```python
from build123d import *

# Parameters (mm, degrees)
SKETCH1_R           = 2
BOSS_EXTRUDE1_DEPTH = 2
SKETCH2_R           = 0.5
BOSS_EXTRUDE2_DEPTH = 12
DOME1_FACE_RADIUS   = 2
DOME1_HEIGHT        = 0.8
CUT_EXTRUDE1_DEPTH  = 3.8
CIRPATTERN1_COUNT   = 40


with BuildPart() as part:
    # Sketch1 → Boss-Extrude1 (new body)
    with BuildSketch(Plane(origin=(0, 0, 0), x_dir=(0, 0, -1), z_dir=(1, 0, 0))):
        Circle(SKETCH1_R)
    extrude(amount=BOSS_EXTRUDE1_DEPTH)

    # Sketch2 → Boss-Extrude2 (add)
    with BuildSketch(Plane(origin=(2, 0, 0), x_dir=(0, 0, -1), z_dir=(1, 0, 0))):
        Circle(SKETCH2_R)
    extrude(amount=BOSS_EXTRUDE2_DEPTH)

    # Dome1: a dome of height H over a round flat face of radius A is a cap of a sphere of radius (A * A + H * H) / (2 * H)
    dome1_r = (DOME1_FACE_RADIUS * DOME1_FACE_RADIUS + DOME1_HEIGHT * DOME1_HEIGHT) / (2 * DOME1_HEIGHT)
    dome1_base = Plane((0, 0, 0), z_dir=(-1, 0, 0))
    with Locations(dome1_base.offset(DOME1_HEIGHT - dome1_r)):
        dome1_ball = Sphere(dome1_r, mode=Mode.PRIVATE)
    add(split(dome1_ball, bisect_by=dome1_base, keep=Keep.TOP, mode=Mode.PRIVATE))

    # Sketch3 → Cut-Extrude1 (cut, through all)
    with BuildSketch(Plane(origin=(2, 0, 0), x_dir=(0, 0, -1), z_dir=(1, 0, 0))):
        with BuildLine():
            Line((-0.005039775, 1.853565527), (0.135996541, 1.995370878))
            ThreePointArc((0.135996541, 1.995370878), (-0.005437904, 1.999992607), (-0.146845126, 1.994601842))
            Line((-0.146845126, 1.994601842), (-0.005039775, 1.853565527))
        make_face()
    cut_extrude1 = extrude(amount=-CUT_EXTRUDE1_DEPTH, mode=Mode.SUBTRACT)

    # CirPattern1: Cut-Extrude1 ×40 about axis
    cirpattern1_axis = Axis((0, 0, 0), (1, 0, 0))
    for i in range(1, CIRPATTERN1_COUNT):
        add(cut_extrude1.rotate(cirpattern1_axis, i * 360 / CIRPATTERN1_COUNT), mode=Mode.SUBTRACT)


solid = part.part
```
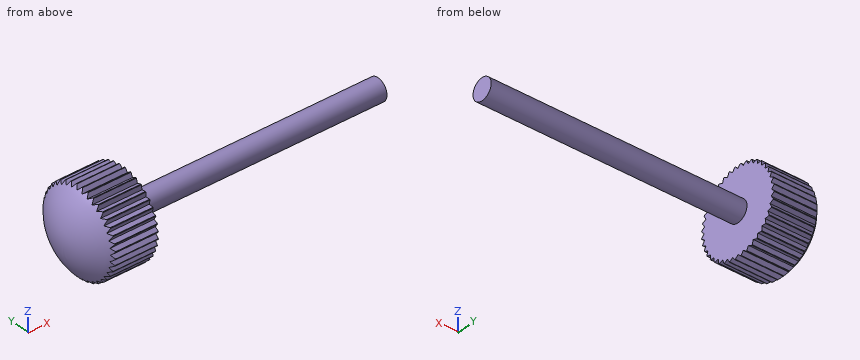
CAD build for the part. Positions are in the model's coordinates, mm. Give positions to 0.01 mm unless a question says otherwise; leave off trailing zeros. Loops run counter-clockwise (first coordinate to the right, second up) from the corner with the lowest first, then second, coordinate; pieces in that order, holes last. Notation, with made-up numbers: M 66,71 L 74,71 A16 cw 74,82 Z; hole C 30.25,84.5 d1. An arc over 180 degrees is marked long. Use one line per item in the form item = value.
Item 1: Drill centre lines: probe 1 along X at (y, z) = (-0.35, -0.1); probe 2 along X at (y, z) = (-0.1, -0.75); probe 3 along Y at (x, z) = (11.25, -0.1). Where is each one in solid material? Low to high. Write a range as from..to.
Determined:
probe_1 = -0.78..14
probe_2 = -0.7..2
probe_3 = -0.49..0.49
Item 2: Flat gauge pins, fed straight in: pin 1 (2 mm diameter, centred on x = 4.5, z = 0, fed in from -Y); pin 2 (2 mm diameter, centred on x = 11.5, z = 1, fed in from +Y); pin 3 (1 mm diameter, centred on y = 0.5, z = 1, fed in from +X); pin 4 (2 mm diameter, centred on y = 0, z = -0.5, fed in from -X). Where does each tip first touch, or does it go through?
Determined:
pin_1 = -0.5
pin_2 = 0.5
pin_3 = 2
pin_4 = -0.8
Item 3: Slice it at A-A (x = 12.5). List the corners of the cut face in (y, z).
Determined:
outline = C 0,0 d1
